Source: three-view drawing plus pictorial views. Frame: mm from the lowest corner of the part. A direction names the side the tool comes from. Give positions to 0.01 mm unless a question says otherwise; leave off trailing zeros. Order: outer loops, then holes, each group sorted by start corner. A loop starts at its lowest first (then second) coordinate and runs counter-clockwise, first axis right, second up. Notation, with made-up numbers: (71.5, 27.5) -> (91.5, 27.5) arc R14 ccw to (91.5, 44.5) -> close; hole circle Ø2 at (67, 77.5). An arc over 180 degrees is marked (long way). Write item = value, one per line.
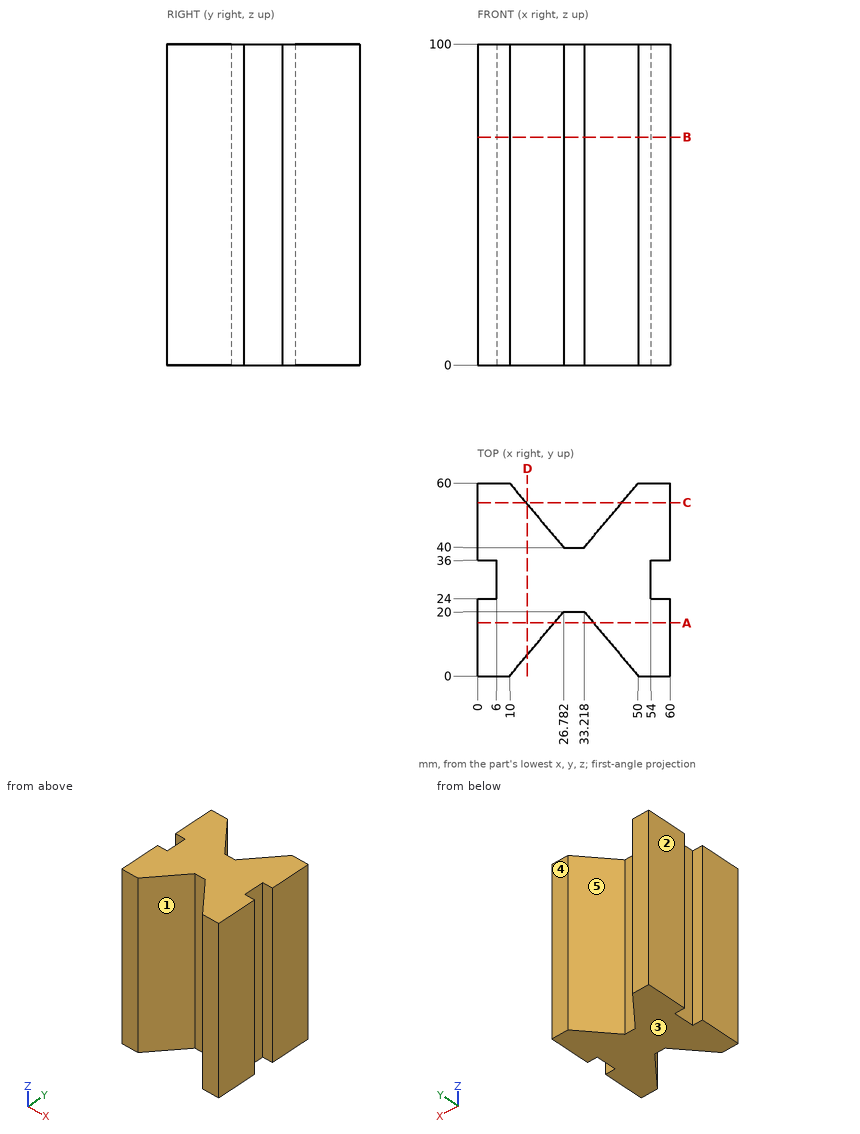
1) Section query A-A (y = 16.5). Output: boundary loops of the cut face in (x, z).
Check sheet entries:
outline = (0, 0) -> (23.85, 0) -> (23.85, 100) -> (0, 100) -> close; (36.15, 0) -> (60, 0) -> (60, 100) -> (36.15, 100) -> close
2) Section query C-C (y = 54). Output: boundary loops of the cut face in (x, z), plus the area to 3 significant figures.
Check sheet entries:
outline = (0, 0) -> (15.03, 0) -> (15.03, 100) -> (0, 100) -> close; (44.97, 0) -> (60, 0) -> (60, 100) -> (44.97, 100) -> close
area = 3,010 mm²
3) Section query D-D (x = 15.5). Output: boundary loops of the cut face in (y, z), plus the area to 3 significant figures.
Check sheet entries:
outline = (6.55, 0) -> (53.45, 0) -> (53.45, 100) -> (6.55, 100) -> close
area = 4,690 mm²
4) First-contact query: P1, Ø7, axis at x = 29, z = 54.5, coming from the -Y side; P2, Ø1, axis at y = 31, z = 12, coming from the -X side; P3, Ø7, axis at x = 30.5, z = 47, coming from the +Y side. Flat tips, straight axial feed; report the tip coordinate or a pass-through.
Check sheet entries:
P1 = 18.47
P2 = 6
P3 = 40.93
5) Section query B-B (z = 71). Output: boundary loops of the cut face in (x, y).
Check sheet entries:
outline = (0, 0) -> (10, 0) -> (26.78, 20) -> (33.22, 20) -> (50, 0) -> (60, 0) -> (60, 24) -> (54, 24) -> (54, 36) -> (60, 36) -> (60, 60) -> (50, 60) -> (33.22, 40) -> (26.78, 40) -> (10, 60) -> (0, 60) -> (0, 36) -> (6, 36) -> (6, 24) -> (0, 24) -> close
6) Line query: line 1 (X direction, y = 13.5, z = 51.5); line 2 (X direction, y = 54.5, z = 48) (3 decimals); line 3 (X direction, y = 25.5, z = 86.5). Output: solid intervals per line, ascending. Write a range as from..to.
Check sheet entries:
line_1 = 0..21.33, 38.67..60
line_2 = 0..14.615, 45.385..60
line_3 = 6..54
7) Mould query, pull axis X, two halves, no side actions, for the marked faces 1, 2 and 3. Classes: +X half, -X half, draft (parallel to the pull), parting line (faces both ways), or undercut.
Check sheet entries:
face_1 = undercut
face_2 = -X half
face_3 = draft
8) Reachability of the marked faces 4 and 5 from +Z, -Z, +X, -X, +Y, -Y: full face, straight path, thin tool, end or side. Return the list, or none.
Check sheet entries:
face_4 = +Z, -Z, +X, -X, +Y
face_5 = +Z, -Z, +Y
